from build123d import *

# Parameters (mm, degrees)
SKETCH1_R           = 7.112045721
BOSS_EXTRUDE1_DEPTH = 2.75
BOSS_EXTRUDE2_DEPTH = 3
BOSS_EXTRUDE3_DEPTH = 2.5


with BuildPart() as part:
    # Sketch1 → Boss-Extrude1 (new body)
    with BuildSketch(Plane(origin=(0, 0, 0), x_dir=(1, 0, 0), z_dir=(0, 1, 0))):
        with BuildLine():
            Line((-35, 86.51875), (35, 86.51875))
            ThreePointArc((35, 86.51875), (38.535533906, 85.054283906), (40, 81.51875))
            Line((40, 81.51875), (40, -81.51875))
            ThreePointArc((40, -81.51875), (38.535533906, -85.054283906), (35, -86.51875))
            Line((35, -86.51875), (-35, -86.51875))
            ThreePointArc((-35, -86.51875), (-38.535533906, -85.054283906), (-40, -81.51875))
            Line((-40, -81.51875), (-40, 81.51875))
            ThreePointArc((-40, 81.51875), (-38.535533906, 85.054283906), (-35, 86.51875))
        make_face()
        with Locations((0, -48.920084539)):
            Circle(SKETCH1_R, mode=Mode.SUBTRACT)
        with BuildLine():
            Line((37, 77.51875), (37, 42.76875))
            ThreePointArc((37, 42.76875), (34, 39.76875), (31, 42.76875))
            Line((31, 42.76875), (31, 77.51875))
            ThreePointArc((31, 77.51875), (34, 80.51875), (37, 77.51875))
        make_face(mode=Mode.SUBTRACT)
        with BuildLine():
            Line((-37, 77.51875), (-37, 42.76875))
            ThreePointArc((-37, 42.76875), (-34, 39.76875), (-31, 42.76875))
            Line((-31, 42.76875), (-31, 77.51875))
            ThreePointArc((-31, 77.51875), (-34, 80.51875), (-37, 77.51875))
        make_face(mode=Mode.SUBTRACT)
        with BuildLine():
            Line((37, -77.51875), (37, -42.76875))
            ThreePointArc((37, -42.76875), (34, -39.76875), (31, -42.76875))
            Line((31, -42.76875), (31, -77.51875))
            ThreePointArc((31, -77.51875), (34, -80.51875), (37, -77.51875))
        make_face(mode=Mode.SUBTRACT)
        with BuildLine():
            Line((-37, -77.51875), (-37, -42.76875))
            ThreePointArc((-37, -42.76875), (-34, -39.76875), (-31, -42.76875))
            Line((-31, -42.76875), (-31, -77.51875))
            ThreePointArc((-31, -77.51875), (-34, -80.51875), (-37, -77.51875))
        make_face(mode=Mode.SUBTRACT)
        with BuildLine():
            Line((37, 24.76875), (37, -27.76875))
            ThreePointArc((37, -27.76875), (34, -30.76875), (31, -27.76875))
            Line((31, -27.76875), (31, 24.76875))
            ThreePointArc((31, 24.76875), (34, 27.76875), (37, 24.76875))
        make_face(mode=Mode.SUBTRACT)
        with BuildLine():
            Line((-37, 24.76875), (-37, -27.76875))
            ThreePointArc((-37, -27.76875), (-34, -30.76875), (-31, -27.76875))
            Line((-31, -27.76875), (-31, 24.76875))
            ThreePointArc((-31, 24.76875), (-34, 27.76875), (-37, 24.76875))
        make_face(mode=Mode.SUBTRACT)
    extrude(amount=BOSS_EXTRUDE1_DEPTH)



with BuildPart() as body_2:
    # Sketch3 → Boss-Extrude2 (new body)
    with BuildSketch(Plane(origin=(0, 12.958063193, 93.198377578), x_dir=(0, -0.990472215, 0.137712714), z_dir=(0, 0.137712714, 0.990472215))):
        with BuildLine():
            Line((-125.30290794, 25), (-60.504073198, 25))
            ThreePointArc((-60.504073198, 25), (-52.018791824, 21.485281374), (-48.504073198, 13))
            Line((-48.504073198, 13), (-48.504073198, -13))
            ThreePointArc((-48.504073198, -13), (-52.018791824, -21.485281374), (-60.504073198, -25))
            Line((-60.504073198, -25), (-225.30290794, -25))
            ThreePointArc((-225.30290794, -25), (-233.788189314, -21.485281374), (-237.30290794, -13))
            Line((-237.30290794, -13), (-237.30290794, 25))
            ThreePointArc((-237.30290794, 25), (-233.788189314, 33.485281374), (-225.30290794, 37))
            Line((-225.30290794, 37), (-147.30290794, 37))
            add(Edge.make_bspline(
                [(-147.30290794, 37), (-144.065512893, 37), (-135.5827842, 31), (-129.980550468, 25), (-125.30290794, 25)],
                knots=[0, 0, 0, 0, 0.5, 1, 1, 1, 1], degree=3))
        make_face()
    extrude(amount=-BOSS_EXTRUDE2_DEPTH)


with BuildPart() as part_1:
    add(part.part)

    add(body_2.part)  # Boss-Extrude3 merges body 2
    # Sketch4 → Boss-Extrude3 (add, symmetric)
    with BuildSketch(Plane(origin=(10, 0, 0), x_dir=(0, 0, -1), z_dir=(1, 0, 0))):
        Polygon((-59.513534896, 233.445335393), (-50.513534896, 232.678056605), (-44.72786756, 85.636126776), (-49.474356372, 2.75), (-81.51875, 2.75), (-82.335595034, 69.302056709), align=None)
    boss_extrude3 = extrude(amount=BOSS_EXTRUDE3_DEPTH, both=True)

    # Mirror1: Boss-Extrude3 across plane
    add(boss_extrude3.mirror(Plane(origin=(0, 0, 0), x_dir=(0, 0, 1), z_dir=(1, 0, 0))))


solid = part_1.part
For this review, take the finished solid that the model builds, in its own axes (mm). A direction names the side the tool comes from. Give positions to 0.01 mm unless a question says otherwise; leave off trailing zeros. Write each loop counter-clockwise with the first axis right and the second up, starting at its lowest first coordinate (ties: lowest second). Pieces come first, ordered by that corner, then holes. Notation, with made-up numbers: (67, 79.5) -> (79, 79.5) arc R21 ccw to (79, 113.5) -> close; hole circle Ø3 at (2.5, -38.5). An arc over 180 degrees is marked (long way). Use CSV: the item, a comma, the result in double quotes.
Q1. Tool access review of faces 5 (the face through (25, 105, 79)), 6 (the face through (10.035, 233.067, 55.077)), 7 (the face through (-7.5, 94, 63)), 8 (the face through (37, 198, 66)): name each direction out of +Z, -Z, +X, -X, +Y, -Y from which nothing blocks a thin tool from reaching the whole face with its end or side.
Conclusion:
face 5,"+Z, -Z, +X"
face 6,"-Z, +X, -X"
face 7,"-Z"
face 8,"+Z, -Z, +X, +Y"
Q2. Take a section at A-A, the plane x = 0. Write out the cut boundary in (y, z), then the cut area to 3 significant figures.
Conclusion:
outline,"(0, -86.52) -> (2.75, -86.52) -> (2.75, 41.81) -> (0, 41.81) -> close; (0, 56.03) -> (2.75, 56.03) -> (2.75, 86.52) -> (0, 86.52) -> close; (60.59, 83.55) -> (247.59, 57.55) -> (248, 60.52) -> (61, 86.52) -> close"
area,"1,000 mm2"
Q3. Mouldability with a two-part tool opening along Y and no side actions: class faces 1 (the face through (-12.5, 94, 63)), 2 (the face through (6.4, 153.2, 73.7)), 3 (the face through (38.5, 1.36, -85.09)), 4 (the face through (6.43, 152.78, 70.73)) as pulls with the +Y half, pulls with the -Y half, needs draft (parallel to the pull), parting line crosses it, or undercut.
Conclusion:
face 1,"undercut"
face 2,"pulls with the +Y half"
face 3,"needs draft"
face 4,"undercut"
Q4. Take a section at C-C, the plane y = 45. Write out the cut boundary in (x, z).
Conclusion:
outline,"(-12.5, 47.05) -> (-7.5, 47.05) -> (-7.5, 82.04) -> (-12.5, 82.04) -> close; (7.5, 47.05) -> (12.5, 47.05) -> (12.5, 82.04) -> (7.5, 82.04) -> close"
Q5. To check wall thickness, follow probe 1 along Z at (x, y) = (0, 1.8); probe 2 along X at (y, z) = (57, 59.5); probe 3 along Y at (x, z) = (-7, -19). State the ranges of each line that lie inside material, in increasing order. Write a range as [from, to].
Conclusion:
probe 1,"[-86.52, 41.81], [56.03, 86.52]"
probe 2,"[-12.5, -7.5], [7.5, 12.5]"
probe 3,"[0, 2.75]"
Q6. For P1, Ø4, axis at y = 192, z = 67, coming from the +X side; P2, Ø1, axis at x = -21.5, y = 72, coming from the -Z side; P3, Ø24, axis at x = -6, z = -25, coming from the +Y side, all flat-tipped, find the tip position at first contact; note any pin that passes through.
Conclusion:
P1,"x = 37"
P2,"z = 81.89"
P3,"y = 2.75"
Q7. Take a section at B-B, the plane z = 8. Write out the cut boundary in (x, y), then the cut area to 3 significant figures.
Conclusion:
outline,"(-40, 0) -> (-37, 0) -> (-37, 2.75) -> (-40, 2.75) -> close; (-31, 0) -> (31, 0) -> (31, 2.75) -> (-31, 2.75) -> close; (37, 0) -> (40, 0) -> (40, 2.75) -> (37, 2.75) -> close"
area,"187 mm2"
